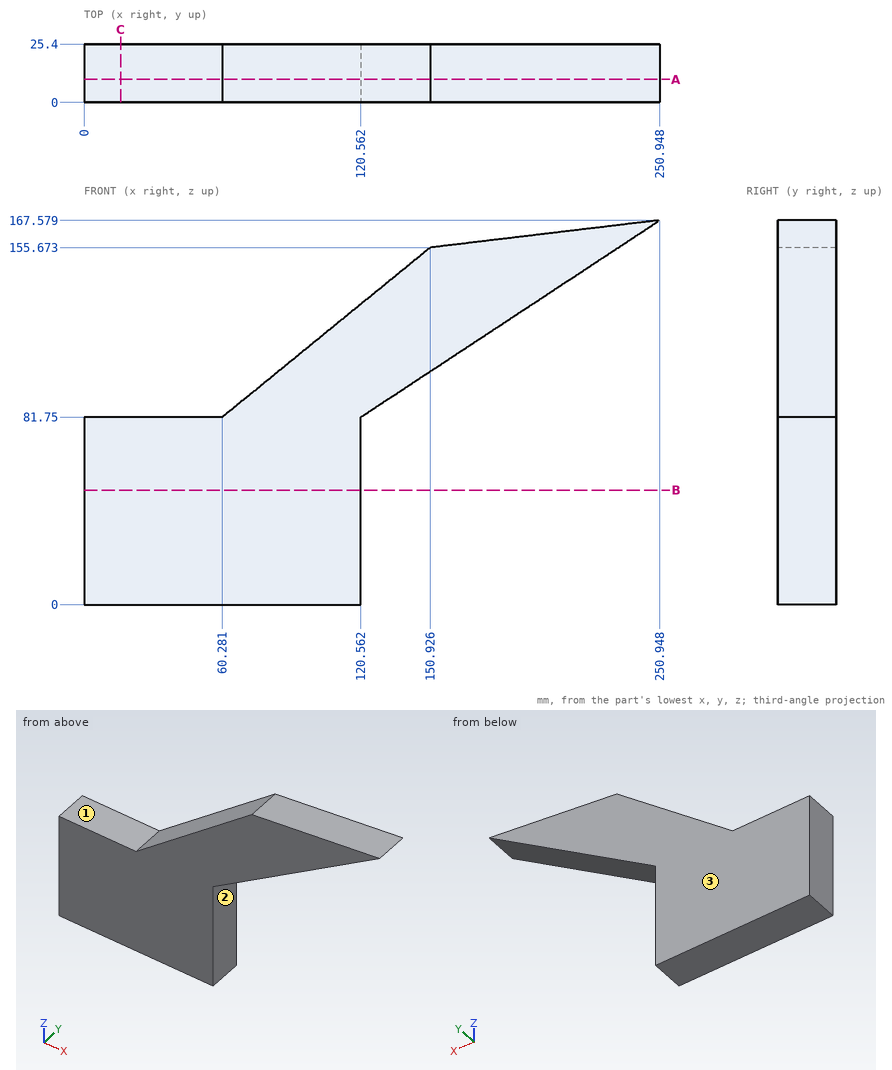
For this review, use the dimensioned drawing (mm, ordinates from the lowest corner) and the shaded views. A direction names the side the tool comes from. Give positions to 0.01 mm unless a question says otherwise; leave off trailing zeros. Order: outer loops, then holes, each group sorted by start corner. A loop starts at its lowest first (then second) coordinate and runs counter-clockwise, first axis right, second up. Notation, with made-up numbers: (33, -32.5) - (45, -32.5) arc R20 cw to (45, -22.5) - close; hole circle Ø11 at (65.5, 79.5). An arc over 180 degrees is marked (long way). Write item = value, one per line. Start each with the question number.
Q1. We need section A-A on y = 10. State the section outline as (x, z) points.
Q2. We need section B-B on z = 50. State the section outline as (x, y) points.
Q3. Tool access review of the marked faces 1, 2 and 3: name each direction out of +Z, -Z, +X, -X, +Y, -Y from which nothing blocks a thin tool from reaching the whole face with its end or side.
Q4. Clearance check with flat-ended pins moving along their axes: pin 1 Ø10 at (x, y) = (148.5, 16.5) entering from +Z; pin 2 Ø5 at (x, y) = (149.5, 13) entering from +Z; pin 3 Ø12.5 at (x, y) = (24.5, 17) entering from +Z. State where each tip first meets the part, or that it passes through.
Q5. To check wall thickness, follow L1, parallel to X at y = 3.75, z = 28.5; L2, parallel to Z at x = 12.5, y = 14.5; L3, parallel to Z at x = 87, y = 14.5. State the ranges of each line that lie inside material, in increasing order. Write a range as from..to.
Q6. We need section C-C on x = 16. State the section outline as (y, z) points.
Working result:
q1.outline = (0, 0) - (120.56, 0) - (120.56, 81.75) - (250.95, 167.58) - (150.93, 155.67) - (60.28, 81.75) - (0, 81.75) - close
q2.outline = (0, 0) - (120.56, 0) - (120.56, 25.4) - (0, 25.4) - close
q3.face_1 = +Z, -X, +Y, -Y
q3.face_2 = -Z, +X, +Y, -Y
q3.face_3 = +Z, -Z, +X, -X, +Y
q4.pin_1 = 155.98
q4.pin_2 = 155.8
q4.pin_3 = 81.75
q5.L1 = 0..120.56
q5.L2 = 0..81.75
q5.L3 = 0..103.54
q6.outline = (0, 0) - (25.4, 0) - (25.4, 81.75) - (0, 81.75) - close
